Check sheet for the modelled part. Datum: model origin and axes. Units: mm. Face numbers are marked on the shaded views. Give positions to 0.01 mm unless a question says otherwise; leave off trailing zeros. Loops run counter-clockwise (first coordinate to the right, second up) from the corner with the lowest first, then second, coordinate; pieces in that order, holes last.
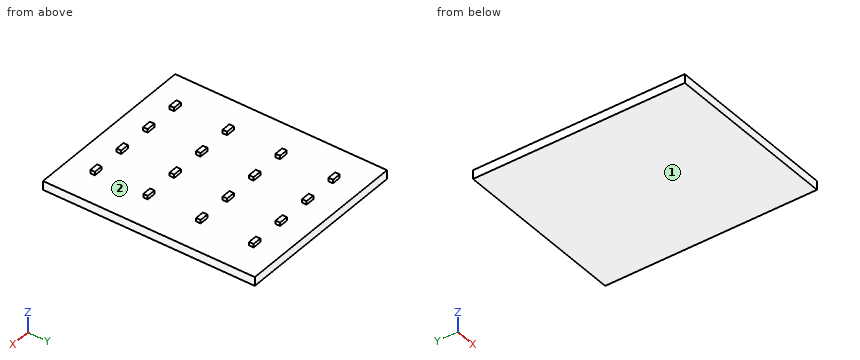
```python
from build123d import *

# Parameters (mm, degrees)
SKETCH_1_W      = 100
SKETCH_1_H      = 120
EXTRUDE_1_DEPTH = 5
SKETCH_2_W      = 5.086017552
SKETCH_2_H      = 2.543008776
EXTRUDE_2_DEPTH = 2


with BuildPart() as part:
    # 草图1 → 凸台-拉伸1 (new body)
    with BuildSketch(Plane.XY):
        Rectangle(SKETCH_1_W, SKETCH_1_H)
    extrude(amount=EXTRUDE_1_DEPTH)

    # 草图2 → 凸台-拉伸2 (add)
    with BuildSketch(Plane.XY.offset(5)):
        with Locations((-10, 45)):
            Rectangle(SKETCH_2_W, SKETCH_2_H)
        with Locations((-30, 45)):
            Rectangle(SKETCH_2_W, SKETCH_2_H)
        with Locations((10, 45)):
            Rectangle(SKETCH_2_W, SKETCH_2_H)
        with Locations((30, 45)):
            Rectangle(SKETCH_2_W, SKETCH_2_H)
        with Locations((-30, 15)):
            Rectangle(SKETCH_2_W, SKETCH_2_H)
        with Locations((-10, 15)):
            Rectangle(SKETCH_2_W, SKETCH_2_H)
        with Locations((10, 15)):
            Rectangle(SKETCH_2_W, SKETCH_2_H)
        with Locations((30, 15)):
            Rectangle(SKETCH_2_W, SKETCH_2_H)
        with Locations((-30, -15)):
            Rectangle(SKETCH_2_W, SKETCH_2_H)
        with Locations((-10, -15)):
            Rectangle(SKETCH_2_W, SKETCH_2_H)
        with Locations((10, -15)):
            Rectangle(SKETCH_2_W, SKETCH_2_H)
        with Locations((30, -15)):
            Rectangle(SKETCH_2_W, SKETCH_2_H)
        with Locations((-30, -45)):
            Rectangle(SKETCH_2_W, SKETCH_2_H)
        with Locations((-10, -45)):
            Rectangle(SKETCH_2_W, SKETCH_2_H)
        with Locations((10, -45)):
            Rectangle(SKETCH_2_W, SKETCH_2_H)
        with Locations((30, -45)):
            Rectangle(SKETCH_2_W, SKETCH_2_H)
    extrude(amount=EXTRUDE_2_DEPTH)


solid = part.part
```
(1) Section check B-B on y = 9.5. Record the boundary of the cut face in (x, z), plus the area to 3 significant figures.
(2) Section check C-C on x = 18. Record the boundary of the cut face in (y, z).
(3) Gauge pin test, flat ends, axial feed: pin 1 Ø0.6 at (y, z) = (-14.5, 6.5) entering from -X; pin 2 Ø1 at (x, z) = (11, 6) entering from +Y; pin 3 Ø1.6 at (x, z) = (-9, 6) entering from -Y. Record the tip position at first contact, or that the pin passes through.
(4) Release check for a two-part mould opening along Y. For the marked faces 1 and 2 record: pulls with the +Y half, pulls with the -Y half, needs draft (parallel to the pull), parting line crosses it, or undercut.
(5) Section check A-A on x = 29.5. Record the boundary of the cut face in (y, z).
(6) Material ranges on line 1 (Z direction, x = 32.5, y = -34), recorded low to high.
Computed values:
1. outline: (-50, 0) - (50, 0) - (50, 5) - (-50, 5) - close
1. area: 500 mm2
2. outline: (-60, 0) - (60, 0) - (60, 5) - (-60, 5) - close
3. pin 1: stops at x = -32.54
3. pin 2: stops at y = 46.27
3. pin 3: stops at y = -46.27
4. face 1: needs draft
4. face 2: undercut
5. outline: (-60, 0) - (60, 0) - (60, 5) - (46.27, 5) - (46.27, 7) - (43.73, 7) - (43.73, 5) - (16.27, 5) - (16.27, 7) - (13.73, 7) - (13.73, 5) - (-13.73, 5) - (-13.73, 7) - (-16.27, 7) - (-16.27, 5) - (-43.73, 5) - (-43.73, 7) - (-46.27, 7) - (-46.27, 5) - (-60, 5) - close
6. line 1: z = 0 to 5
